```python
from build123d import *

# Parameters (mm, degrees)
F0_W     = 21.825
F0_H     = 6.35
F0_W_2   = 6.35
F0_H_2   = 21.825
F1_DEPTH = 25
F2_SIZE  = 1
F3_R     = 1


with BuildPart() as f1:
    # F0 (on Top) → F1 (new body)
    with BuildSketch(Plane.XY):
        with Locations((-14.0875, 0)):
            Rectangle(F0_W, F0_H)
        Rectangle(F0_W_2, F0_H)
        with Locations((14.0875, 0)):
            Rectangle(F0_W, F0_H)
        with Locations((0, 14.0875)):
            Rectangle(F0_W_2, F0_H_2)
    extrude(amount=F1_DEPTH)

    # F2
    f2_edges = [f1.edges().sort_by_distance(p)[0] for p in [
        (-25, 0, 0),
        (0, -3.175, 0),
        (25, 0, 0),
        (14.0875, 3.175, 0),
        (3.175, 14.0875, 0),
        (0, 25, 0),
        (-3.175, 14.0875, 0),
        (-14.0875, 3.175, 0),
        (-25, 0, 25),
        (0, -3.175, 25),
        (25, 0, 25),
        (14.0875, 3.175, 25),
        (3.175, 14.0875, 25),
        (0, 25, 25),
        (-3.175, 14.0875, 25),
        (-14.0875, 3.175, 25),
    ]]
    chamfer(f2_edges, length=F2_SIZE)

    # F3
    f3_edges = [f1.edges().sort_by_distance(p)[0] for p in [
        (3.175, 3.175, 12.5),
        (-3.175, 3.175, 12.5),
    ]]
    fillet(f3_edges, radius=F3_R)


solid = f1.part
```
Part model, mm, in its own coordinate system. A direction names the side the tool comes from. Coordinates: 2 decimals unless noted, no trailing zeros. Write each loop counter-clockwise with the first axis right and the second up, starting at its lowest first coordinate (ties: lowest second). Pieces come first, ordered by that corner, then holes.
Item 1: Slice it at C-C (z = 21.25). Write the cut outline in (x, y) (3 decimals).
Item 2: Probe line 1 (Y direction, x = 22, z = 1.75) (3 decimals); line 2 (Z direction, x = 2.5, y = 23.25) (3 decimals). List the from-to ranges inside material, lowest first.
Item 3: Pin check, flat tips, straight feed: pin 1 (10.5 mm diameter, centred on y = 14.5, z = 9.5, fed in from +X) (3 decimals); pin 2 (10.5 mm diameter, centred on x = 17.5, z = 15, fed in from +Y) (3 decimals); pin 3 (12 mm diameter, centred on x = 8, y = 8, fed in from +Z); pin 4 (1 mm diameter, centred on y = 18.5, z = 4.5, fed in from -X) (3 decimals). Stop position of each tip, or through.
Item 4: Slice it at A-A (y = 6.25). Write the cut outline in (x, z) (3 decimals), and give its area (3 significant figures).
Item 5: Which spindle directions (+Z, -Z, +X, -X, +Y, -Y) get a long thin tool onto all of the face, cutting with end or side? Do faces 1 (the face through (15, 3.175, 12)), 2 (the face through (-2.669, 13.428, 24.506)), 3 (the face through (2.669, 13.428, 0.494)), 4 (the face through (2.669, 13.428, 24.506)), 5 (the face through (-3.175, 14, 12)). Say none if no direction does.
Results found:
1. outline: (-25, -3.175) - (25, -3.175) - (25, 3.175) - (4.175, 3.175) arc R1 cw to (3.175, 4.175) - (3.175, 25) - (-3.175, 25) - (-3.175, 4.175) arc R1 cw to (-4.175, 3.175) - (-25, 3.175) - close
2. line 1: y = -3.175 to 3.175
2. line 2: z = 0.325 to 24.675
3. pin 1: stops at x = 3.175
3. pin 2: stops at y = 3.175
3. pin 3: stops at z = 25
3. pin 4: stops at x = -3.175
4. outline: (-3.175, 1) - (-2.175, 0) - (2.175, 0) - (3.175, 1) - (3.175, 24) - (2.175, 25) - (-2.175, 25) - (-3.175, 24) - close
4. area: 157 mm2
5. face 1: +Z, -Z, +X, +Y
5. face 2: +Z, -X, +Y
5. face 3: -Z, +X, +Y
5. face 4: +Z, +X, +Y
5. face 5: +Z, -Z, -X, +Y
